from build123d import *

# Parameters (mm, degrees)
F0_W     = 72.644
F0_H     = 72.644
F1_DEPTH = 228.6
F2_W     = 19.05
F2_H     = 11.684
F2_W_2   = 11.684
F2_H_2   = 19.05
F3_DEPTH = 228.601
F4_R     = 2.38125
F5_DEPTH = 19.05
F6_R     = 2.38125
F7_DEPTH = 19.05


with BuildPart() as f1:
    # F0 (on Top) → F1 (new body)
    with BuildSketch(Plane.XY):
        with Locations((36.322, 36.322)):
            Rectangle(F0_W, F0_H)
    extrude(amount=F1_DEPTH)

    # F2 (on face) → F3 (cut, through all)
    with BuildSketch(Plane.XY.offset(228.6)):
        with Locations((9.525, 36.322)):
            Rectangle(F2_W, F2_H)
        with Locations((36.322, 9.525)):
            Rectangle(F2_W_2, F2_H_2)
    extrude(amount=-F3_DEPTH, mode=Mode.SUBTRACT)

    # F4 (on face) → F5 (join, through all)
    with BuildSketch(Plane.XZ.offset(-19.05)):
        with Locations((36.322, 12.7)):
            Circle(F4_R)
    extrude(amount=F5_DEPTH)

    # F6 (on face) → F7 (join, through all)
    with BuildSketch(Plane(origin=(19.05, 0, 0), x_dir=(0, -1, 0), z_dir=(-1, 0, 0))):
        with Locations((-36.322, 12.7)):
            Circle(F6_R)
    extrude(amount=F7_DEPTH)


solid = f1.part
For this review, take the finished solid that the model builds, in its own axes (mm). A direction names the side the tool comes from. Coordinates: 2 decimals unless noted, no trailing zeros. Loops run counter-clockwise (first coordinate to the right, second up) from the corner with the lowest first, then second, coordinate; pieces in that order, holes last. Notation, with made-up numbers: (-34.5, 0.5) -> (-24.5, 0.5) arc R18 cw to (-24.5, 34.5) -> close; hole circle Ø3 at (68.25, 72.5). An arc over 180 degrees is marked (long way). Write each question's results on one line, items separated by ' | '.
Q1. Add section A-A, the plane x = 14.5. State the section outline as (y, z) points, then the cut area to 3 significant figures.
Taken from the geometry:
outline: (0, 0) -> (30.48, 0) -> (30.48, 228.6) -> (0, 228.6) -> close; circle Ø4.76 at (36.32, 12.7); (42.16, 0) -> (72.64, 0) -> (72.64, 228.6) -> (42.16, 228.6) -> close | area: 14,000 mm²
Q2. Mouldability with a two-part tool opening along Y and no side actions: class faces 5 (the flat face through (0, 15, 113)), 6 (the flat face through (15, 0, 113)), 7 (the flat face through (9, 42.164, 116)), 8 (the flat face through (36, 72.644, 113)) as +Y half, -Y half, draft (parallel to the pull), parting line (faces both ways), or undercut.
Taken from the geometry:
face 5: draft | face 6: -Y half | face 7: undercut | face 8: +Y half
Q3. Machinability: for faces 1 (the cylindrical face through (33.943, 9.658, 12.805)), 2 (the cylindrical face through (9.66, 34.12, 11.79)), 3 (the flat face through (9, 30.48, 116)), 4 (the flat face through (30.48, 9, 116)), which of the approach directions +Z, -Z, +X, -X, +Y, -Y give a long, thin tool a straight path to every point of the face, cutting with its end or side? Answer none if there is none.
Taken from the geometry:
face 1: -Y | face 2: -X | face 3: +Z, -Z, -X | face 4: +Z, -Z, -Y
Q4. For pin 1 Ø9.5 at (x, z) = (34.5, 58) entering from -Y; pin 2 Ø9.5 at (y, z) = (35.5, 80.5) entering from -X, all flat-tipped, find the tip position at first contact; note any pin that passes through.
Taken from the geometry:
pin 1: y = 0 | pin 2: x = 19.05
Q5. Add section C-C, the plane z = 12.7. State the section outline as (x, y) points.
Taken from the geometry:
outline: (0, 0) -> (30.48, 0) -> (30.48, 19.05) -> (33.94, 19.05) -> (33.94, 0) -> (38.7, 0) -> (38.7, 19.05) -> (42.16, 19.05) -> (42.16, 0) -> (72.64, 0) -> (72.64, 72.64) -> (0, 72.64) -> (0, 42.16) -> (19.05, 42.16) -> (19.05, 38.7) -> (0, 38.7) -> (0, 33.94) -> (19.05, 33.94) -> (19.05, 30.48) -> (0, 30.48) -> close
Q6. To check wall thickness, follow line 1 along X through (y, z) = (18, 21.5); line 2 along Y through (x, z) = (38, 116.5). State the ranges of each line that lie inside material, in increasing order. Write a range as [from, to].
Taken from the geometry:
line 1: [0, 30.48], [42.16, 72.64] | line 2: [19.05, 72.64]
Q7. Add section D-D, the plane z = 41. State the section outline as (x, y) points.
Taken from the geometry:
outline: (0, 0) -> (30.48, 0) -> (30.48, 19.05) -> (42.16, 19.05) -> (42.16, 0) -> (72.64, 0) -> (72.64, 72.64) -> (0, 72.64) -> (0, 42.16) -> (19.05, 42.16) -> (19.05, 30.48) -> (0, 30.48) -> close
